```python
from build123d import *

# Parameters (mm, degrees)
SKETCH1_W           = 10.16
SKETCH1_H           = 41.275
SKETCH1_W_2         = 91.44
SKETCH1_H_2         = 10.16
BOSS_EXTRUDE1_DEPTH = 10.16


with BuildPart() as part:
    # Sketch1 → Boss-Extrude1 (new body)
    with BuildSketch(Plane.XY):
        Polygon((193.04, -10.16), (101.6, -10.16), (10.16, -10.16), (10.16, -51.435), (10.16, -92.71), (650.24, -92.71), (650.24, -51.435), (650.24, -10.16), (558.8, -10.16), (467.36, -10.16), (375.92, -10.16), (284.48, -10.16), align=None)
        with Locations((655.32, -72.0725)):
            Rectangle(SKETCH1_W, SKETCH1_H)
        with Locations((604.52, -5.08)):
            Rectangle(SKETCH1_W_2, SKETCH1_H_2)
        with Locations((421.64, -5.08)):
            Rectangle(SKETCH1_W_2, SKETCH1_H_2)
        with Locations((238.76, -5.08)):
            Rectangle(SKETCH1_W_2, SKETCH1_H_2)
        with Locations((55.88, -5.08)):
            Rectangle(SKETCH1_W_2, SKETCH1_H_2)
        with Locations((5.08, -72.0725)):
            Rectangle(SKETCH1_W, SKETCH1_H)
    extrude(amount=BOSS_EXTRUDE1_DEPTH)


solid = part.part
```
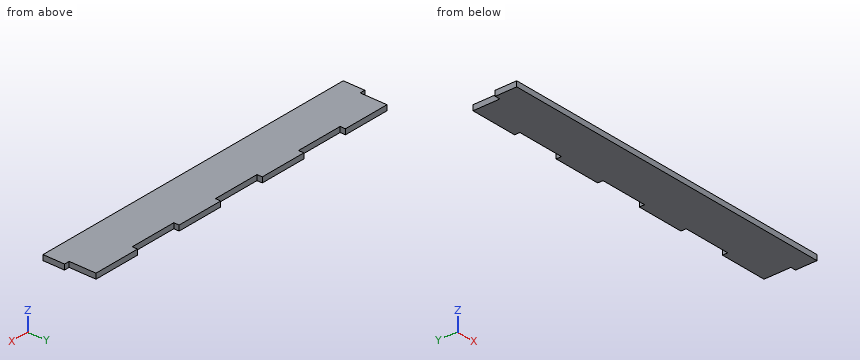
Geometry: final body of the model. Coordinates: model frame, mm. Coordinates: 2 decimals unless noted, no trailing zeros. Order: outer loops, then holes, each group sorted by start corner. A loop starts at its lowest first (then second) coordinate and runs counter-clockwise, first axis right, second up. Notation, with made-up numbers: (-7, -16) - (37, -16) arc R14 cw to (37, 9) - close; hole circle Ø10 at (-16, 71.25). An arc over 180 degrees is marked (long way). Return JSON: item names as keys, results as strings. Group by question number.
1. Cut plane B-B (x = 494). Output: boundary loops of the cut face in (y, z), plus the area to 3 significant figures.
2. Material intervals for line 1 along X through (y, z) = (-8.5, 5); line 2 along Y through (x, z) = (154, 2.25); line 3 along X through (y, z) = (-31, 4), sorted ascending. Write a range as [from, to].
3. Pin query (flat end, axial travel): pin 1 (5 mm diameter, centred on y = -3.5, z = 6.5, fed in from +X); pin 2 (3 mm diameter, centred on y = -4, z = 7.5, fed in from -X); pin 3 (3 mm diameter, centred on x = 6, z = 5, fed in from +Y) (3 decimals). Return the tip coordinate at first contact, or that it passes through.
4. Cut plane A-A (z = 4). Output: boundary loops of the cut face in (x, y) (3 decimals), plus the area to 3 significant figures.
5. Cut plane C-C (y = -32). Output: boundary loops of the cut face in (x, z), plus the area to 3 significant figures.
Resolved:
{
 "1": {"outline": "(-92.71, 0) - (-10.16, 0) - (-10.16, 10.16) - (-92.71, 10.16) - close", "area": "839 mm²"},
 "2": {"line 1": "x = [10.16, 101.6], [193.04, 284.48], [375.92, 467.36], [558.8, 650.24]", "line 2": "y = [-92.71, -10.16]", "line 3": "x = [10.16, 650.24]"},
 "3": {"pin 1": "stops at x = 650.24", "pin 2": "stops at x = 10.16", "pin 3": "stops at y = -51.435"},
 "4": {"outline": "(0, -92.71) - (660.4, -92.71) - (660.4, -51.435) - (650.24, -51.435) - (650.24, 0) - (558.8, 0) - (558.8, -10.16) - (467.36, -10.16) - (467.36, 0) - (375.92, 0) - (375.92, -10.16) - (284.48, -10.16) - (284.48, 0) - (193.04, 0) - (193.04, -10.16) - (101.6, -10.16) - (101.6, 0) - (10.16, 0) - (10.16, -51.435) - (0, -51.435) - close", "area": "57,400 mm²"},
 "5": {"outline": "(10.16, 0) - (650.24, 0) - (650.24, 10.16) - (10.16, 10.16) - close", "area": "6,500 mm²"}
}
